Autodesk Inventor part; units mm, degrees
ref_plane "YZ Plane" through (0, 0, 0) normal (1, 0, 0) x (0, 1, 0)
ref_plane "XZ Plane" through (0, 0, 0) normal (0, 1, 0) x (-1, 0, 0)
ref_plane "XY Plane" through (0, 0, 0) normal (0, 0, 1) x (1, 0, 0)
sketch "Sketch1" plane through (0, 0, 0) normal (0, 0, 1) x (1, 0, 0)
  line L0 (-8.25, 0) -> (8.25, 0)
  line L1 (-8.25, 0) -> (-8.25, 1)
  line L2 (-8.25, 1) -> (-6.75, 1)
  line L3 (-6.75, 1) -> (-6.75, 1.25)
  line L4 (-6.75, 1.25) -> (-5.5, 1.25)
  line L5 (-5.5, 1.25) -> (-5.5, 1.25)
  line L6 (-5, 0.95) -> (1.5, 0.95)
  line L7 (1.5, 0.95) -> (1.5, 1.75)
  line L8 (1.5, 1.75) -> (6, 1.75)
  line L9 (6, 1.75) -> (6, 1.25)
  line L10 (6, 1.25) -> (6.75, 1.25)
  line L11 (6.75, 1.25) -> (6.75, 1)
  line L12 (6.75, 1) -> (8.25, 1)
  line L13 (8.25, 1) -> (8.25, 0)
  line L14 (0, 0) -> (0, 3.0708) construction
  line L15 (-5.5, 1.25) -> (-5.5, 1.75)
  line L16 (-5.5, 1.75) -> (-5, 1.75)
  line L17 (-5, 1.75) -> (-5, 0.95)
  dimension "d0" = 2
  dimension "d1" = 16.5
  dimension "d2" = 1.5
  dimension "d3" = 1.5
  dimension "d4" = 2.5
  dimension "d5" = 3.5
  dimension "d6" = 1.9
  dimension "d12" = 7
  dimension "d13" = 0.75
  dimension "d14" = 0.5
  dimension "d16" = 3.5
  dimension "d17" = 1.75
revolve "Revolution1" add sketch "Sketch1" angle 360 about axis through (-8.25, 0, 0) along (1, 0, 0)
sketch "Sketch2" plane through (8.25, 0, 0) normal (1, 0, 0) x (0, 0, -1)
  circle A0 centre (0, 0) radius 1.75
  line L0 (-1.5811, 0.75) -> (1.5811, 0.75)
  dimension "d9" = 0.75
extrude "Extrusion1" cut sketch "Sketch2" against normal up to surface (6.75 mm away) contours L0 A0 picked at (0, 1.0833)
properties part number "MCP axle" material "Stainless Steel"
Read the model definition and answer for the solid it produces. Units are mm, in the model's axes. A direction names the side the tool comes from. Give positions to 0.01 mm unless a question says otherwise; leave off trailing zeros. Loops run counter-clockwise (first coordinate to the right, second up) from the corner with the lowest first, then second, coordinate; pieces in that order, holes last. Notation, with made-up numbers: (-12, -38.75) -> (9, -38.75) arc R25 cw to (9, -11.75) -> close; hole circle Ø9 at (14, 62.5). An arc over 180 degrees is marked (long way). Answer as CSV lines item,"result".
Item 1: Determine the mould class of faces 6 (the face through (-5.5, 1, -1)), 7 (the face through (4, 0.75, 0)), 8 (the face through (1.5, -1.1, 0)) for opening direction X: +X half, -X half, draft (parallel to the pull), parting line (faces both ways), or undercut.
Returned:
face 6,"-X half"
face 7,"draft"
face 8,"undercut"
Item 2: Find section C-C on x = -5.25. Give the vertices of the cut face in (y, z), plus the area to 3 significant figures.
Returned:
outline,"circle Ø3.5 at (0, 0)"
area,"9.62 mm²"
Item 3: Consider line 1 (X direction, y = -0.3, z = -1.3); line 2 (X direction, y = 0.95, z = -0.7); line 3 (X direction, y = 1.1, z = -0.95). Determine where each line is inside the solid, lowest interval first. Write a range as [from, to].
Returned:
line 1,"x = [-5.5, -5], [1.5, 6]"
line 2,"x = [-6.75, -5]"
line 3,"x = [-5.5, -5]"
Item 4: This flat-tipped pin is pushed along its axis until it touches: pin 1 (0.9 mm diameter, centred on x = 3.5, z = 0, fed in from +Y). Where does it stop, or does it pass through?
Returned:
pin 1,"stops at y = 0.75"
Item 5: Find section A-A on z = 0. Give the vertices of the cut face in (x, y), plus the area to 3 significant figures.
Returned:
outline,"(-8.25, -1) -> (-6.75, -1) -> (-6.75, -1.25) -> (-5.5, -1.25) -> (-5.5, -1.75) -> (-5, -1.75) -> (-5, -0.95) -> (1.5, -0.95) -> (1.5, -1.75) -> (6, -1.75) -> (6, -1.25) -> (6.75, -1.25) -> (6.75, -1) -> (8.25, -1) -> (8.25, 0.75) -> (1.5, 0.75) -> (1.5, 0.95) -> (-5, 0.95) -> (-5, 1.75) -> (-5.5, 1.75) -> (-5.5, 1.25) -> (-6.75, 1.25) -> (-6.75, 1) -> (-8.25, 1) -> close"
area,"35.6 mm²"
Item 6: Find section D-D on x = -3.25. Give the vertices of the cut face in (y, z).
Returned:
outline,"circle Ø1.9 at (0, 0)"
Item 7: Find section B-B on y = 0. Give the vertices of the cut face in (x, z), plus the area to 4 significant figures.
Returned:
outline,"(-8.25, -1) -> (-6.75, -1) -> (-6.75, -1.25) -> (-5.5, -1.25) -> (-5.5, -1.75) -> (-5, -1.75) -> (-5, -0.95) -> (1.5, -0.95) -> (1.5, -1.75) -> (6, -1.75) -> (6, -1.25) -> (6.75, -1.25) -> (6.75, -1) -> (8.25, -1) -> (8.25, 1) -> (6.75, 1) -> (6.75, 1.25) -> (6, 1.25) -> (6, 1.75) -> (1.5, 1.75) -> (1.5, 0.95) -> (-5, 0.95) -> (-5, 1.75) -> (-5.5, 1.75) -> (-5.5, 1.25) -> (-6.75, 1.25) -> (-6.75, 1) -> (-8.25, 1) -> close"
area,"40.85 mm²"
Item 8: For faces 1 (the face through (8.25, 0, 0)), 2 (the face through (-6.12, -0.27, -1.22)), 3 (the face through (-5, 1, -1)), 4 (the face through (6.38, -1.25, 0.04)), 5 (the face through (-8.25, 0, 0)), determine the directions among +Z, -Z, +X, -X, +Y, -Y from which every point of the face is accessible in a straight line to the end or side of a thin tool.
Returned:
face 1,"+Z, -Z, +X, +Y, -Y"
face 2,"-X"
face 3,"none"
face 4,"+X"
face 5,"+Z, -Z, -X, +Y, -Y"
